Read the model definition and answer for the solid it produces. Units are mm, in the model's axes. A direction names the side the tool comes from. Give positions to 0.01 mm unless a question says otherwise; leave off trailing zeros. Order: outer loops, then holes, each group sorted by start corner. A loop starts at its lowest first (then second) coordinate and runs counter-clockwise, first axis right, second up. Notation, with made-up numbers: (-26, 67.25) - (17, 67.25) arc R19 cw to (17, 91.25) - close; hole circle Ø7 at (77.25, 62). An arc over 180 degrees is marked (long way). Return JSON: item names as keys, results as strings.
```python
from build123d import *

# Parameters (mm, degrees)
F0_W     = 700
F0_H     = 500
F1_DEPTH = 300
F2_W     = 5
F2_H     = 34.9
F3_DEPTH = 266.7
F4_W     = 233.9330434799
F4_H     = 17.4498
F5_DEPTH = 25.4


with BuildPart() as f1:
    # F0 (on Front) → F1 (new body)
    with BuildSketch(Plane.XZ):
        with Locations((-350, -250)):
            Rectangle(F0_W, F0_H)
    extrude(amount=F1_DEPTH)

    # F2 (on face) → F3 (join)
    with BuildSketch(Plane.XZ.offset(300)):
        with Locations((-350, -334.2865335016)):
            Rectangle(F2_W, F2_H)
    extrude(amount=F3_DEPTH)

    # F4 (on face) → F5 (cut)
    with BuildSketch(Plane(origin=(-352.5, 0, 0), x_dir=(0, -1, 0), z_dir=(-1, 0, 0))):
        with Locations((416.96652174, -325.5614335016)):
            Rectangle(F4_W, F4_H)
        Polygon((533.9330434799, -316.8365335016), (566.7, -351.7365335016), (566.7, -316.8365335016), align=None)
    extrude(amount=-F5_DEPTH, mode=Mode.SUBTRACT)


solid = f1.part
```
Q1. A cutting plane is placed at B-B (z = -69.5). Write down the section's boundary in (x, y), and give its area (3 significant figures).
Values:
{"outline": "(-700, -300) - (0, -300) - (0, 0) - (-700, 0) - close", "area": "210,000 mm²"}
Q2. A cutting plane is placed at A-A (y = -518.5). Write down the section's boundary in (x, z).
Values:
{"outline": "(-352.5, -351.74) - (-347.5, -351.74) - (-347.5, -334.29) - (-352.5, -334.29) - close"}
Q3. Given pin 1 (5.5 mm diameter, centred on x = -349.5, y = -429, fed in from +Z); pin 2 (1.5 mm diameter, centred on x = -349, y = -426.5, fed in from -Z); pin 3 (10.5 mm diameter, centred on y = -411.5, z = -340.5, fed in from -X), each flat-ended and moving along its own axis, determine where each tip first touches the part or whether it passes through.
Values:
{"pin 1": "stops at z = -334.29", "pin 2": "stops at z = -351.74", "pin 3": "stops at x = -352.5"}
Q4. Consider L1, parallel to X at y = -439.5, z = -349.5; L2, parallel to Y at x = -250, z = -191.5. Determine where each line is inside the solid, lowest interval first.
Values:
{"L1": "x = -352.5 to -347.5", "L2": "y = -300 to 0"}
Q5. For faces 1 (the flat face through (-355, 0, -246)), 2 (the flat face through (-352.5, -431, -342)), 3 (the flat face through (-347.5, -431, -342)), determine the directions among +Z, -Z, +X, -X, +Y, -Y from which every point of the face is accessible in a straight line to the end or side of a thin tool.
Values:
{"face 1": "+Z, -Z, +X, -X, +Y", "face 2": "+Z, -Z, -X, -Y", "face 3": "+Z, -Z, +X, -Y"}
